from build123d import *

# Parameters (mm, degrees)
F0_W     = 23.6728
F0_H     = 15.7734
F1_DEPTH = 4.7625
F2_R     = 2.4257
F3_DEPTH = 1.7526
F4_W     = 20.6248
F4_H     = 13.2334
F7_DEPTH = 8.3058
F5_R     = 3.2258
F8_DEPTH = 8.3058
F6_R     = 2.3876
F9_DEPTH = 8.3058


with BuildPart() as f1:
    # F0 (on Top) → F1 (new body, symmetric)
    with BuildSketch(Plane.XY):
        Rectangle(F0_W, F0_H)
    extrude(amount=F1_DEPTH, both=True)

    # F2 (on face) → F3 (join)
    with BuildSketch(Plane.XY.offset(4.7625)):
        with Locations((-7.9883, 3.9751)):
            Circle(F2_R)
        with Locations((0, 3.9624)):
            Circle(F2_R)
        with Locations((7.9883, 3.9624)):
            Circle(F2_R)
        with Locations((7.9883, -3.9624)):
            Circle(F2_R)
        with Locations((0, -3.9624)):
            Circle(F2_R)
        with Locations((-7.9883, -3.9751)):
            Circle(F2_R)
    extrude(amount=F3_DEPTH)

    # F4 (on face) → F7 (cut)
    with BuildSketch(Plane(origin=(0, 0, -4.7625), x_dir=(1, 0, 0), z_dir=(0, 0, -1))):
        Rectangle(F4_W, F4_H)
    extrude(amount=-F7_DEPTH, mode=Mode.SUBTRACT)

    # F5 (on face) → F8 (join)
    with BuildSketch(Plane(origin=(0, 0, -4.7625), x_dir=(1, 0, 0), z_dir=(0, 0, -1))):
        with Locations((-3.5306, 0)):
            Circle(F5_R)
        with Locations((3.5306, 0)):
            Circle(F5_R)
    extrude(amount=-F8_DEPTH)

    # F6 (on face) → F9 (cut)
    with BuildSketch(Plane(origin=(0, 0, -4.7625), x_dir=(1, 0, 0), z_dir=(0, 0, -1))):
        with Locations((-3.5306, 0)):
            Circle(F6_R)
        with Locations((3.5306, 0)):
            Circle(F6_R)
    extrude(amount=-F9_DEPTH, mode=Mode.SUBTRACT)


solid = f1.part
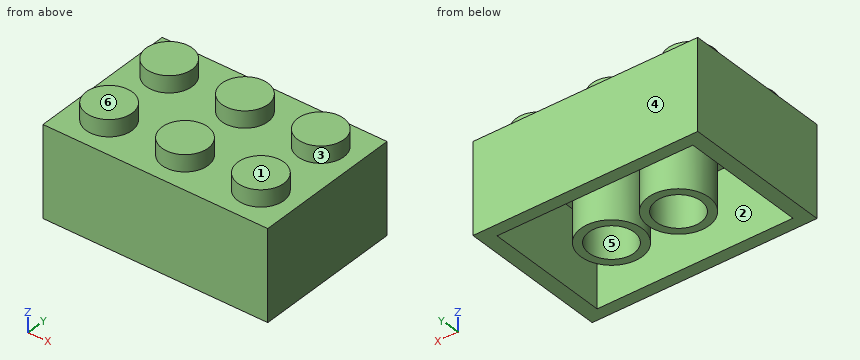
Work out the finished part from the listing and answer in its coordinate system (mm). Face numbers are marked on the shaded views. A direction names the side the tool comes from. Round coordinates to 2 decimals unless told otherwise and drop trailing zeros. Loops run counter-clockwise (first coordinate to the right, second up) from the corner with the lowest first, then second, coordinate; pieces in that order, holes last. Notation, with made-up numbers: (32, -22.75) - (90, -22.75) arc R29 ccw to (90, 2.25) - close; hole circle Ø5 at (62.25, 5). An arc over 180 degrees is marked (long way). One line per item, written item: value.
Q1. Find section B-B on x = 0. Give the vertices of the cut face in (y, z).
Check values:
outline: (-7.89, -4.76) - (-6.62, -4.76) - (-6.62, 3.54) - (6.62, 3.54) - (6.62, -4.76) - (7.89, -4.76) - (7.89, 4.76) - (6.39, 4.76) - (6.39, 6.52) - (1.54, 6.52) - (1.54, 4.76) - (-1.54, 4.76) - (-1.54, 6.52) - (-6.39, 6.52) - (-6.39, 4.76) - (-7.89, 4.76) - close
Q2. Find section C-C on y = -3.5. Give the vertices of the cut face in (x, z).
Check values:
outline: (-11.84, -4.76) - (-10.31, -4.76) - (-10.31, 3.54) - (10.31, 3.54) - (10.31, -4.76) - (11.84, -4.76) - (11.84, 4.76) - (10.37, 4.76) - (10.37, 6.52) - (5.61, 6.52) - (5.61, 4.76) - (2.38, 4.76) - (2.38, 6.52) - (-2.38, 6.52) - (-2.38, 4.76) - (-5.61, 4.76) - (-5.61, 6.52) - (-10.37, 6.52) - (-10.37, 4.76) - (-11.84, 4.76) - close
Q3. Find section A-A on z = -2.5. Give the vertices of the cut face in (x, y).
Check values:
outline: (-11.84, -7.89) - (11.84, -7.89) - (11.84, 7.89) - (-11.84, 7.89) - close; circle Ø6.45 at (-3.53, 0); circle Ø6.45 at (3.53, 0); hole (-10.31, -6.62) - (10.31, -6.62) - (10.31, 6.62) - (-10.31, 6.62) - close; hole circle Ø4.78 at (-3.53, 0); hole circle Ø4.78 at (3.53, 0)
Q4. The mould has two halves that part along Y. Classify the marked faces 4, 5 and 6: +Y half, -Y half, draft (parallel to the pull), parting line (faces both ways), or undercut.
Check values:
face 4: +Y half
face 5: undercut
face 6: draft
Q5. For the marked faces 1, 2 and 3, determine the directions among +Z, -Z, +X, -X, +Y, -Y from which every point of the face is accessible in a straight line to the end or side of a thin tool.
Check values:
face 1: +Z, +X, -X, +Y, -Y
face 2: -Z
face 3: +Z
Q6. Straight lines are drawn through the part: probe 1 along X at (y, z) = (0, 0.75); probe 2 along Y at (x, z) = (3.5, 0.25); probe 3 along Y at (x, z) = (-4, -2.5). For each, find the intervals that lie inside material, in ascending order.
Check values:
probe 1: -11.84 to -10.31, -6.76 to -5.92, -1.14 to -0.3, 0.3 to 1.14, 5.92 to 6.76, 10.31 to 11.84
probe 2: -7.89 to -6.62, -3.23 to -2.39, 2.39 to 3.23, 6.62 to 7.89
probe 3: -7.89 to -6.62, -3.19 to -2.34, 2.34 to 3.19, 6.62 to 7.89
Q7. Each of these flat-tipped pins is pushed along its axis until it touches: pin 1 Ø8 at (x, y) = (-4.5, -4) entering from +Z; pin 2 Ø4 at (x, y) = (-3.53, 0) entering from -Z. Where does it stop, or does it pass through?
Check values:
pin 1: z = 6.52
pin 2: z = 3.54
Q8. Find section D-D on z = 6. Give the vertices of the cut face in (x, y), and give its area (3 significant figures).
Check values:
outline: circle Ø4.85 at (-7.99, -3.98); circle Ø4.85 at (-7.99, 3.98); circle Ø4.85 at (0, -3.96); circle Ø4.85 at (0, 3.96); circle Ø4.85 at (7.99, -3.96); circle Ø4.85 at (7.99, 3.96)
area: 111 mm2
